Check sheet for the drawn part. Datum: minimum x, y, z corner. Units: mm. Coordinates: 2 decimals unless noted, no trailing zeros. Loops run counter-clockwise (first coordinate to the right, second up) from the corner with the lowest first, then second, coordinate; pieces in that order, holes last.
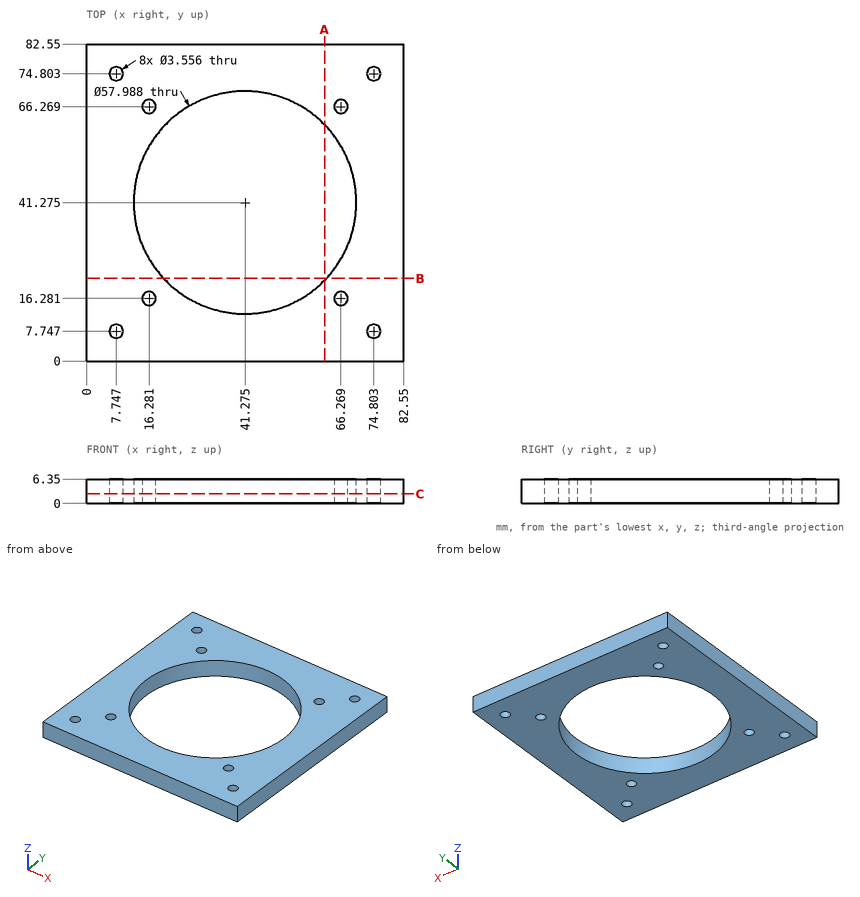
(1) Sectioned sample at C-C on z = 2.5. State how many separate pieces and enclosed holes the cut face has, and give its area (3 significant figures).
Findings:
separate pieces: 1
enclosed holes: 9
area: 4,090 mm2
(2) Sectioned sample at B-B on y = 21.5. Record the cut outline in (x, z).
Findings:
outline: (0, 0) - (20.07, 0) - (20.07, 6.35) - (0, 6.35) - close; (62.48, 0) - (82.55, 0) - (82.55, 6.35) - (62.48, 6.35) - close
(3) Sectioned sample at A-A on x = 62. Record the cut outline in (y, z).
Findings:
outline: (0, 0) - (21, 0) - (21, 6.35) - (0, 6.35) - close; (61.55, 0) - (82.55, 0) - (82.55, 6.35) - (61.55, 6.35) - close
(4) Scan lines: L1, parallel to Y at x = 51, z = 0.75; L2, parallel to X at y = 64, z = 2.5; L3, parallel to Y at x = 41.5, z = 1. Record each from-to range of solid material in increasing order.
Findings:
L1: y = 0 to 13.96, 68.59 to 82.55
L2: x = 0 to 23.27, 59.28 to 82.55
L3: y = 0 to 12.28, 70.27 to 82.55
